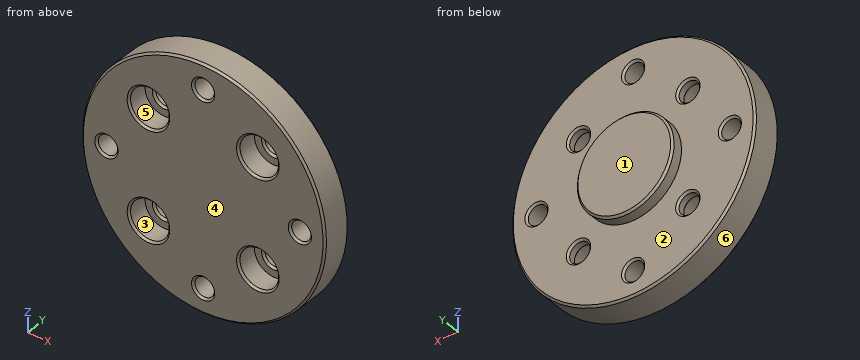
```python
from build123d import *

# Parameters (mm, degrees)
SKETCH1_R                                           = 31.5
BOSS_EXTRUDE1_DEPTH                                 = 8
SKETCH30_R                                          = 12.5
BOSS_EXTRUDE3_DEPTH                                 = 3
TAP_DRILL_FOR_M6_TAP3_D                             = 5
CBORE_FOR_M5_HEX_SOCKET_HEAD_CAP_SCREW1_D           = 5.3
CBORE_FOR_M5_HEX_SOCKET_HEAD_CAP_SCREW1_CBORE_D     = 10
CBORE_FOR_M5_HEX_SOCKET_HEAD_CAP_SCREW1_CBORE_DEPTH = 5.4
CHAMFER1_SIZE                                       = 0.5


with BuildPart() as part:
    # Sketch1 → Boss-Extrude1 (new body)
    with BuildSketch(Plane(origin=(0, 0, 0), x_dir=(1, 0, 0), z_dir=(0, 1, 0))):
        with Locations(Location((0, 0, 0), (0, 0, 270))):
            Circle(SKETCH1_R)
    extrude(amount=BOSS_EXTRUDE1_DEPTH)

    # Sketch30 → Boss-Extrude3 (add)
    with BuildSketch(Plane(origin=(0, 8, 0), x_dir=(1, 0, 0), z_dir=(0, 1, 0))):
        with Locations(Location((0, 0, 0), (0, 0, 270))):
            Circle(SKETCH30_R)
    extrude(amount=BOSS_EXTRUDE3_DEPTH)

    # Tap Drill for M6 Tap3 (through all)
    with Locations(Plane(origin=(0, 8, 0), x_dir=(1, 0, 0), z_dir=(0, 1, 0))):
        with Locations((0, -25), (-25, 0), (0, 25), (25, 0)):
            Hole(TAP_DRILL_FOR_M6_TAP3_D / 2)

    # CBORE for M5 Hex Socket Head Cap Screw1 (through all)
    with Locations(Plane(origin=(0, 0, 0), x_dir=(-1, 0, 0), z_dir=(0, -1, 0))):
        with Locations((-14.142135624, 14.142135624), (14.142135624, 14.142135624), (14.142135624, -14.142135624), (-14.142135624, -14.142135624)):
            CounterBoreHole(CBORE_FOR_M5_HEX_SOCKET_HEAD_CAP_SCREW1_D / 2, CBORE_FOR_M5_HEX_SOCKET_HEAD_CAP_SCREW1_CBORE_D / 2, CBORE_FOR_M5_HEX_SOCKET_HEAD_CAP_SCREW1_CBORE_DEPTH)

    # Chamfer1
    chamfer1_edges = [part.edges().sort_by_distance(p)[0] for p in [
        (2.5, 8, 25),
        (2.5, 0, 25),
        (0, 0, -31.5),
        (27.5, 8, 0),
        (27.5, 0, 0),
        (2.5, 8, -25),
        (2.5, 0, -25),
        (-22.5, 8, 0),
        (-22.5, 0, 0),
        (0, 8, -31.5),
        (19.142135624, 0, 14.142135624),
        (11.492135624, 8, 14.142135624),
        (11.492135624, 5.4, 14.142135624),
        (-9.142135624, 0, 14.142135624),
        (-16.792135624, 8, 14.142135624),
        (-16.792135624, 5.4, 14.142135624),
        (-9.142135624, 0, -14.142135624),
        (-16.792135624, 8, -14.142135624),
        (-16.792135624, 5.4, -14.142135624),
        (19.142135624, 0, -14.142135624),
        (11.492135624, 8, -14.142135624),
        (11.492135624, 5.4, -14.142135624),
        (0, 11, -12.5),
    ]]
    chamfer(chamfer1_edges, length=CHAMFER1_SIZE)


solid = part.part
```
Geometry check sheet. Reference: the model listing, model coordinates, mm. Face numbers are marked on the shaded views. A direction names the side the tool comes from. Give positions to 0.01 mm unless a question says otherwise; leave off trailing zeros. Order: outer loops, then holes, each group sorted by start corner. A loop starts at its lowest first (then second) coordinate and runs counter-clockwise, first axis right, second up.
1. Section check A-A, the plane z = 0. Give the number of separate pieces and of enclosed holes in the cut face, and give its area (3 significant figures).
2. Section check C-C, the plane y = 9. Enter the section's corners in (x, z).
3. Access from +Z, -Z, +X, -X, +Y, -Y to the whole of each face (thin tool, end or side, straight path). Record for the marked faces 1, 2 and 3.
4. Thickness scan on L1, parallel to X at y = 5, z = 0; L2, parallel to X at y = 2.5, z = 14; L3, parallel to X at y = 4, z = -25. Record the ranges inside material, lowest first.
5. Release check for a two-part mould opening along X. For the marked faces 4, 5 and 6 record: pulls with the +X half, pulls with the -X half, needs draft (parallel to the pull), parting line crosses it, or undercut.
6. Gauge pin test, flat ends, axial feed: pin 1 Ø8 at (x, z) = (-14.14, -14.14) entering from +Y; pin 2 Ø6 at (x, z) = (14.14, 14.14) entering from -Y; pin 3 Ø6 at (x, z) = (14.14, -14.14) entering from +Y; pin 4 Ø4 at (x, z) = (-25, 0) entering from -Y. Record the tip position at first contact, or that the pin passes through.
Values follow:
1. separate pieces: 3
1. enclosed holes: 0
1. area: 497 mm2
2. outline: circle Ø25 at (0, 0)
3. face 1: +Z, -Z, +X, -X, +Y
3. face 2: +Y
3. face 3: -Y
4. L1: x = -31.5 to -27.5, -22.5 to 22.5, 27.5 to 31.5
4. L2: x = -28.22 to -19.14, -9.14 to 9.14, 19.14 to 28.22
4. L3: x = -19.16 to -2.5, 2.5 to 19.16
5. face 4: needs draft
5. face 5: undercut
5. face 6: parting line crosses it
6. pin 1: stops at y = 8
6. pin 2: stops at y = 5.55
6. pin 3: stops at y = 7.85
6. pin 4: passes through
